```python
from build123d import *

# Parameters (mm, degrees)
SKETCH_1_W          = 60
SKETCH_1_H          = 30
EXTRUDE_1_DEPTH     = 30
SKETCH_2_W          = 60
SKETCH_2_H          = 30
CUT_EXTRUDE_1_DEPTH = 12
SKETCH_3_R          = 1.5
CUT_EXTRUDE_2_DEPTH = 47.086874487


with BuildPart() as part:
    # 草图1 → 凸台-拉伸1 (new body)
    with BuildSketch(Plane.XY):
        Rectangle(SKETCH_1_W, SKETCH_1_H)
    extrude(amount=EXTRUDE_1_DEPTH)

    # 草图2 → 切除-拉伸1 (cut)
    with BuildSketch(Plane.XZ.offset(15)):
        with Locations((0, 15)):
            Rectangle(SKETCH_2_W, SKETCH_2_H)
    extrude(amount=-CUT_EXTRUDE_1_DEPTH, mode=Mode.SUBTRACT)

    # 草图3 → 切除-拉伸2 (cut, through all)
    with BuildSketch(Plane(origin=(0, 15, 0), x_dir=(1, 0, 0), z_dir=(0, 1, 0))):
        with Locations(Location((-27.02081528, -2.97918472, 0), (0, 0, 270))):
            Circle(SKETCH_3_R)
        with Locations(Location((-2.97918472, -2.97918472, 0), (0, 0, 270))):
            Circle(SKETCH_3_R)
        with Locations(Location((-2.97918472, -27.02081528, 0), (0, 0, 270))):
            Circle(SKETCH_3_R)
        with Locations(Location((-27.02081528, -27.02081528, 0), (0, 0, 270))):
            Circle(SKETCH_3_R)
        with Locations(Location((27.02081528, -27.02081528, 0), (0, 0, 90))):
            Circle(SKETCH_3_R)
        with Locations(Location((2.97918472, -27.02081528, 0), (0, 0, 90))):
            Circle(SKETCH_3_R)
        with Locations(Location((2.97918472, -2.97918472, 0), (0, 0, 90))):
            Circle(SKETCH_3_R)
        with Locations(Location((27.02081528, -2.97918472, 0), (0, 0, 90))):
            Circle(SKETCH_3_R)
    extrude(amount=-CUT_EXTRUDE_2_DEPTH, mode=Mode.SUBTRACT)


solid = part.part
```
Design review of the part built by this model. Coordinates are the model's own, in mm. Give positions to 0.01 mm unless a question says otherwise; leave off trailing zeros. Loops run counter-clockwise (first coordinate to the right, second up) from the corner with the lowest first, then second, coordinate; pieces in that order, holes last. Notation, with made-up numbers: M 79,14 L 119,14 A30 ccw 119,49 Z; hole C 54,51.5 d4. An arc over 180 degrees is marked long. Return JSON: item names as keys, results as strings. Group by question number.
Item 1: We need section B-B (z = 26.25). Give the boundary of the cut face in (x, y), and give its area (3 significant figures).
Item 2: We need section A-A (y = 6). Give the number of separate pieces and of enclosed holes in the cut face, and give its area (3 significant figures).
Item 3: For probe 1 along Z at (x, y) = (2.5, -0.5), list the stretches that pass through material, from the lowest coordinate up.
Item 4: Insertion check: pin 1 Ø5 at (x, z) = (-2.98, 27.02) entering from +Y; pin 2 Ø2.5 at (x, z) = (2.98, 27.02) entering from +Y. Each pin has a flat end and moves straight along its axis. Give the tip position at first contact, or say it passes through.
Item 5: Mouldability with a two-part tool opening along X and no side actions: class faces 1 (the flat face through (-30, 6, 15)), 2 (the flat face through (0, 6, 0)), 3 (the cylindrical face through (2.91, 6.13, 28.52)) as released by +X, released by -X, zero draft, split by the parting line, or undercut.
Output:
{
 "1": {"outline": "M -30,-3 L -28.31,-3 L -28.31,15 L -30,15 Z; M -25.73,-3 L -4.27,-3 L -4.27,15 L -25.73,15 Z; M -1.69,-3 L 1.69,-3 L 1.69,15 L -1.69,15 Z; M 4.27,-3 L 25.73,-3 L 25.73,15 L 4.27,15 Z; M 28.31,-3 L 30,-3 L 30,15 L 28.31,15 Z", "area": "895 mm^2"},
 "2": {"separate pieces": "1", "enclosed holes": "8", "area": "1,740 mm^2"},
 "3": {"probe 1": "z = 0 to 1.56, 4.4 to 25.6, 28.44 to 30"},
 "4": {"pin 1": "stops at y = 15", "pin 2": "passes through"},
 "5": {"face 1": "released by -X", "face 2": "zero draft", "face 3": "undercut"}
}
